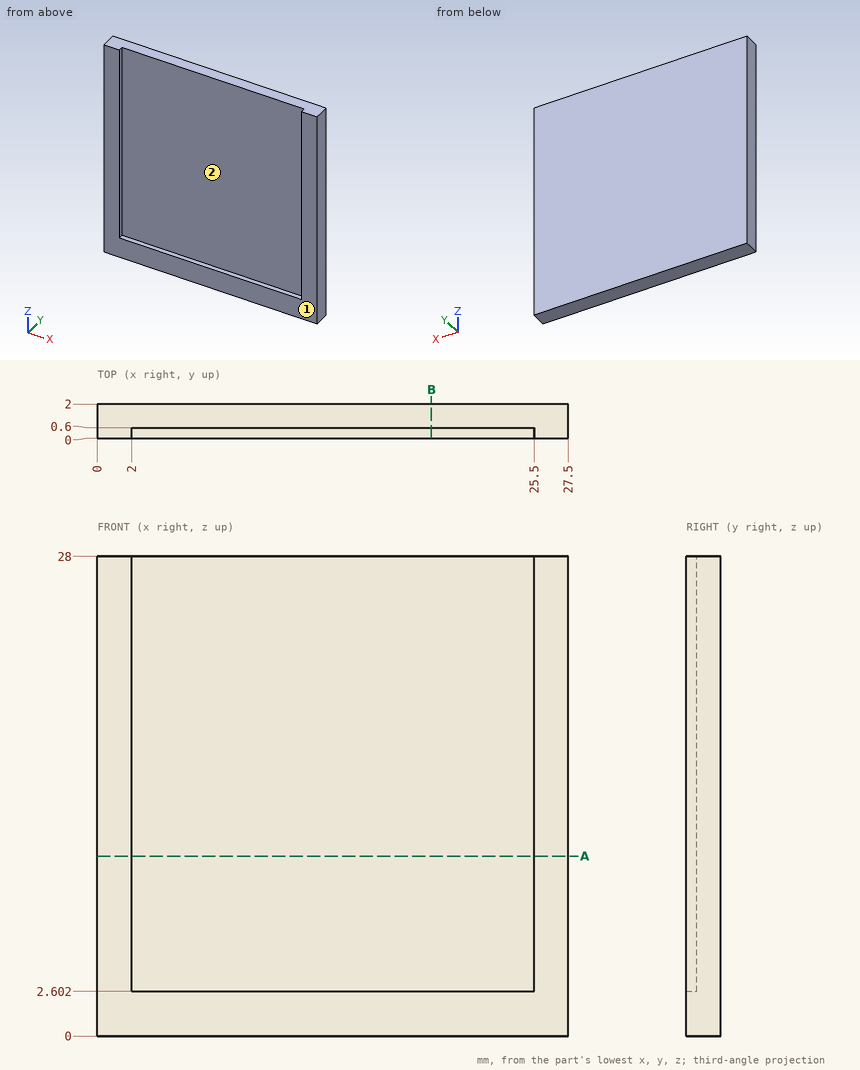
Geometry check sheet. Reference: drawing and pictorial views, mm from the part's lowest x, y, z. Give positions to 0.01 mm unless a question says otherwise; leave off trailing zeros. Order: outer loops, then holes, each group sorted by start corner. A loop starts at its lowest first (then second) coordinate and runs counter-clockwise, first axis right, second up. Notation, with made-up numbers: M 70.25,72 L 94.25,72 A7 ccw 94.25,77 Z; hole C 81,1.5 d4. An arc over 180 degrees is marked long. Answer in a Markdown table with one row per item. Add a question column.
Item 1: Section check A-A, the plane z = 10.5. Enter the section's corners in (x, y), and give its area (3 significant figures).
Item 2: Mould release check, pull along X, two halves, no side actions. Record for the marked faces 1 and 2: released by +X, released by -X, zero draft, split by the parting line, or undercut.
Item 3: Section check B-B, the plane x = 19.5. Enter the section's corners in (y, z).
Item 4: Gauge pin test, flat end, axial feed: pin 1 (10 mm diameter, centred on x = 15, z = 21.5, fed in from -Y). Record the tip position at first contact, or that the pin passes through.
Item 5: Scan lines: probe 1 along X at (y, z) = (0.5, 25.5); probe 2 along Y at (x, z) = (7.5, 26.5); probe 3 along Z at (x, y) = (25, 0.45). Record each from-to range of solid material in increasing order. Write a range as from..to.
Filled sheet:
| question | item | result |
|---|---|---|
| 1 | outline | M 0,0 L 2,0 L 2,0.6 L 25.5,0.6 L 25.5,0 L 27.5,0 L 27.5,2 L 0,2 Z |
| 1 | area | 40.9 mm^2 |
| 2 | face 1 | zero draft |
| 2 | face 2 | undercut |
| 3 | outline | M 0,0 L 2,0 L 2,28 L 0.6,28 L 0.6,2.6 L 0,2.6 Z |
| 4 | pin 1 | stops at y = 0.6 |
| 5 | probe 1 | x = 0..2, 25.5..27.5 |
| 5 | probe 2 | y = 0.6..2 |
| 5 | probe 3 | z = 0..2.6 |
